```python
from build123d import *

# Parameters (mm, degrees)
SKETCH1_W           = 431.8
SKETCH1_H           = 215.9
BOSS_EXTRUDE1_DEPTH = 57.15
SKETCH2_R           = 25.4
BOSS_EXTRUDE2_DEPTH = 3.175


with BuildPart() as part:
    # Sketch1 → Boss-Extrude1 (new body)
    with BuildSketch(Plane(origin=(0, 0, 0), x_dir=(1, 0, 0), z_dir=(0, 1, 0))):
        Rectangle(SKETCH1_W, SKETCH1_H)
    extrude(amount=BOSS_EXTRUDE1_DEPTH)

    # Sketch2 → Boss-Extrude2 (add)
    with BuildSketch(Plane.XZ):
        with Locations(Location((-177.8, 69.85, 0), (0, 0, 270))):
            Circle(SKETCH2_R)
        with Locations(Location((-177.8, -69.85, 0), (0, 0, 270))):
            Circle(SKETCH2_R)
        with Locations(Location((177.8, -69.85, 0), (0, 0, 270))):
            Circle(SKETCH2_R)
        with Locations(Location((177.8, 69.85, 0), (0, 0, 270))):
            Circle(SKETCH2_R)
    extrude(amount=BOSS_EXTRUDE2_DEPTH)


solid = part.part
```
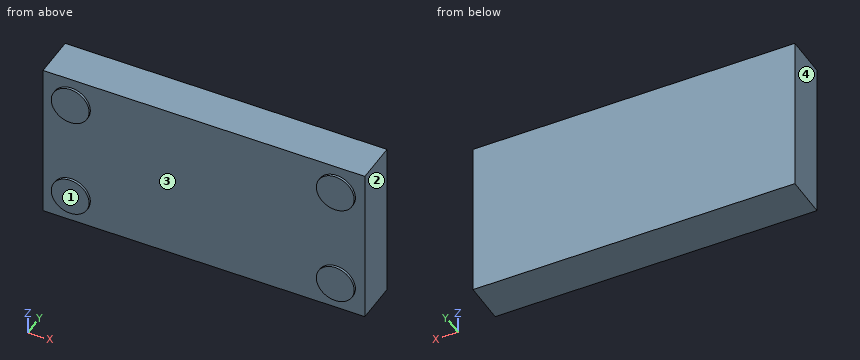
Geometry check sheet. Reference: the model listing, model coordinates, mm. Face numbers are marked on the shaded views. Coordinates: 2 decimals unless noted, no trailing zeros. Loops run counter-clockwise (first coordinate to the right, second up) from the corner with the lowest first, then second, coordinate; pieces in that order, holes last. Notation, with made-up numbers: (24.5, 23) - (76.5, 23) arc R21 cw to (76.5, 36) - close; hole circle Ø7 at (1, 64.25). An arc over 180 degrees is marked (long way). One line per item, written item: value. Start each with the question number.
(1) Cross-section at D-D on z = 35. Enter the section's corners in (x, y), plus the area to 3 significant figures.
(2) Cross-section at B-B on z = -69.85. Enter the section's corners in (x, y) (3 decimals), plus the area to 3 significant figures.
(3) Cross-section at C-C on x = -4.5. Enter the section's corners in (y, z).
(4) Depth check by flat-ended pin: P1, Ø8, axis at x = 11.5, z = -49.5, coming from the -Y side. Enter the tip coordinate at first touch or a pass-through.
(5) Material ranges on line 1 (Y direction, x = -113.5, z = -97), recorded low to high. Write a range as [from, to].
(6) Mould release check, pull along X, two halves, no side actions. Record for the marked faces 1, 2, 3 and 4: released by +X, released by -X, zero draft, split by the parting line, or undercut.
(7) Cross-section at A-A on x = -177.8. Enter the section's corners in (y, z) (3 decimals), plus the area to 3 significant figures.
Results below:
1. outline: (-215.9, 0) - (215.9, 0) - (215.9, 57.15) - (-215.9, 57.15) - close
1. area: 24,700 mm2
2. outline: (-215.9, 0) - (-203.2, 0) - (-203.2, -3.175) - (-152.4, -3.175) - (-152.4, 0) - (152.4, 0) - (152.4, -3.175) - (203.2, -3.175) - (203.2, 0) - (215.9, 0) - (215.9, 57.15) - (-215.9, 57.15) - close
2. area: 25,000 mm2
3. outline: (0, -107.95) - (57.15, -107.95) - (57.15, 107.95) - (0, 107.95) - close
4. P1: stops at y = 0
5. line 1: y = [0, 57.15]
6. face 1: zero draft
6. face 2: released by +X
6. face 3: undercut
6. face 4: released by -X
7. outline: (-3.175, -95.25) - (0, -95.25) - (0, -107.95) - (57.15, -107.95) - (57.15, 107.95) - (0, 107.95) - (0, 95.25) - (-3.175, 95.25) - (-3.175, 44.45) - (0, 44.45) - (0, -44.45) - (-3.175, -44.45) - close
7. area: 12,700 mm2
